```python
from build123d import *

# Parameters (mm, degrees)
BOSS_EXTRUDE1_DEPTH = 3.175
SKETCH2_W           = 156.972
SKETCH2_H           = 22.225
SKETCH2_R           = 4.7625
SKETCH2_R_2         = 0.79375
BOSS_EXTRUDE2_DEPTH = 3.175
FILLET2_R           = 1.27


with BuildPart() as part:
    # Sketch1 → Boss-Extrude1 (new body)
    with BuildSketch(Plane(origin=(0, 0, 0), x_dir=(1, 0, 0), z_dir=(0, 1, 0))):
        Polygon((-78.486, 49.784), (-78.486, 45.72), (-56.261, 45.72), (-56.261, -45.72), (-78.486, -45.72), (-78.486, -49.784), (78.486, -49.784), (78.486, -45.72), (56.261, -45.72), (56.261, 45.72), (78.486, 45.72), (78.486, 49.784), align=None)
    extrude(amount=BOSS_EXTRUDE1_DEPTH)

    # Sketch2 → Boss-Extrude2 (add)
    with BuildSketch(Plane.XY.offset(49.784)):
        with Locations((0, -7.9375)):
            Rectangle(SKETCH2_W, SKETCH2_H)
        with Locations((-67.3735, -7.9375)):
            Circle(SKETCH2_R, mode=Mode.SUBTRACT)
        with Locations(Location((67.3735, -7.9375, 0), (0, 0, 180))):
            Circle(SKETCH2_R, mode=Mode.SUBTRACT)
        with Locations((-47.0535, -12.7)):
            Circle(SKETCH2_R_2, mode=Mode.SUBTRACT)
        with Locations((-37.5285, -12.7)):
            Circle(SKETCH2_R_2, mode=Mode.SUBTRACT)
        with Locations(Location((37.5285, -12.7, 0), (0, 0, 180))):
            Circle(SKETCH2_R_2, mode=Mode.SUBTRACT)
        with Locations(Location((47.0535, -12.7, 0), (0, 0, 180))):
            Circle(SKETCH2_R_2, mode=Mode.SUBTRACT)
    boss_extrude2 = extrude(amount=-BOSS_EXTRUDE2_DEPTH)

    # Mirror2: Boss-Extrude2 across plane
    add(boss_extrude2.mirror(Plane.XY))

    # Fillet2
    # the kernel refuses this fillet: 1.27 mm, written as the material it takes off along each edge
    with BuildSketch(Plane(origin=(-56.261, 0, 45.72), x_dir=(0, 1, 0), z_dir=(-1, 0, 0)), Plane(origin=(56.261, 0, -45.72), x_dir=(0, 1, 0), z_dir=(1, 0, 0)), Plane(origin=(81.514756964, 0, 45.72), x_dir=(0, 1, 0), z_dir=(-1, 0, 0))) as fillet2_piece_1:
        with BuildLine():
            CenterArc((1.211502786, -1.27), FILLET2_R, 90, 72.542396876)
            Line((0, -0.889), (-0.024230056, -0.88138))
            ThreePointArc((-0.024230056, -0.88138), (-0.0254, -0.4445), (-0.0254, 0))
            Line((-0.0254, 0), (0, 0.0254))
            Line((0, 0.0254), (1.211502786, 0.0254))
            Line((1.211502786, 0.0254), (1.211502786, 0))
        make_face()
    extrude(amount=25.253756964, mode=Mode.SUBTRACT)
    with BuildSketch(Plane(origin=(-81.514756964, 0, -45.72), x_dir=(0, 0, -1), z_dir=(1, 0, 0))) as fillet2_piece_2:
        with BuildLine():
            CenterArc((1.27, 1.211502786), FILLET2_R, 180, 72.542396876)
            Line((0, 1.211502786), (-0.0254, 1.211502786))
            Line((-0.0254, 1.211502786), (-0.0254, 0))
            Line((-0.0254, 0), (0, -0.0254))
            ThreePointArc((0, -0.0254), (0.4445, -0.0254), (0.88138, -0.024230056))
            Line((0.88138, -0.024230056), (0.889, 0))
        make_face()
    extrude(amount=25.253756964, mode=Mode.SUBTRACT)
    with BuildSketch(Plane(origin=(81.661, 3.175, 45.72), x_dir=(0, -1, 0), z_dir=(-1, 0, 0)), Plane(origin=(56.261, 3.175, -45.72), x_dir=(0, -1, 0), z_dir=(1, 0, 0)), Plane(origin=(-81.661, 3.175, -45.72), x_dir=(0, -1, 0), z_dir=(1, 0, 0)), Plane(origin=(-56.261, 3.175, 45.72), x_dir=(0, -1, 0), z_dir=(-1, 0, 0))) as fillet2_piece_3:
        with BuildLine():
            CenterArc((FILLET2_R, FILLET2_R), FILLET2_R, 180, 90)
            Line((0, FILLET2_R), (-FILLET2_R * 0.02, FILLET2_R))
            Line((-FILLET2_R * 0.02, FILLET2_R), (-FILLET2_R * 0.02, -FILLET2_R * 0.02))
            Line((-FILLET2_R * 0.02, -FILLET2_R * 0.02), (FILLET2_R, -FILLET2_R * 0.02))
            Line((FILLET2_R, -FILLET2_R * 0.02), (FILLET2_R, 0))
        make_face()
    extrude(amount=25.4, mode=Mode.SUBTRACT)
    with BuildSketch(Plane(origin=(-81.661, -19.05, -46.609), x_dir=(0, 0, -1), z_dir=(1, 0, 0)), Plane(origin=(-81.661, -19.05, -49.784), x_dir=(0, 1, 0), z_dir=(1, 0, 0)), Plane(origin=(-81.661, 3.175, 49.784), x_dir=(0, -1, 0), z_dir=(1, 0, 0)), Plane(origin=(81.661, 3.175, -49.784), x_dir=(0, -1, 0), z_dir=(-1, 0, 0))) as fillet2_piece_4:
        with BuildLine():
            CenterArc((FILLET2_R, FILLET2_R), FILLET2_R, 180, 90)
            Line((0, FILLET2_R), (-FILLET2_R * 0.02, FILLET2_R))
            Line((-FILLET2_R * 0.02, FILLET2_R), (-FILLET2_R * 0.02, -FILLET2_R * 0.02))
            Line((-FILLET2_R * 0.02, -FILLET2_R * 0.02), (FILLET2_R, -FILLET2_R * 0.02))
            Line((FILLET2_R, -FILLET2_R * 0.02), (FILLET2_R, 0))
        make_face()
    extrude(amount=163.322, mode=Mode.SUBTRACT)
    with BuildSketch(Plane(origin=(-81.661, -19.05, 46.609), x_dir=(0, 0, 1), z_dir=(1, 0, 0)), Plane(origin=(-81.661, -19.05, 49.784), x_dir=(0, 1, 0), z_dir=(1, 0, 0))) as fillet2_piece_5:
        with BuildLine():
            CenterArc((FILLET2_R, -FILLET2_R), FILLET2_R, 90, 90)
            Line((0, -FILLET2_R), (-FILLET2_R * 0.02, -FILLET2_R))
            Line((-FILLET2_R * 0.02, -FILLET2_R), (-FILLET2_R * 0.02, FILLET2_R * 0.02))
            Line((-FILLET2_R * 0.02, FILLET2_R * 0.02), (FILLET2_R, FILLET2_R * 0.02))
            Line((FILLET2_R, FILLET2_R * 0.02), (FILLET2_R, 0))
        make_face()
    extrude(amount=163.322, mode=Mode.SUBTRACT)


solid = part.part
```
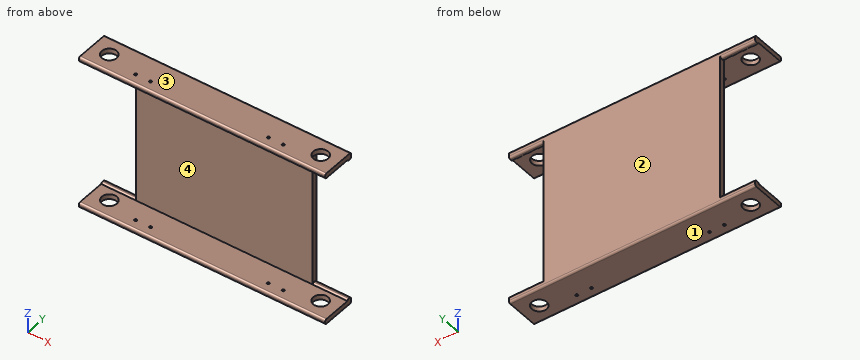
Geometry: final body of the model. Coordinates: model frame, mm. Face numbers are marked on the shaded views. Coordinates: 2 decimals unless noted, no trailing zeros. Order: outer loops, then holes, each group sorted by start corner. A loop starts at its lowest first (then second) coordinate and runs counter-clockwise, first axis right, second up. Notation, with made-up numbers: (22.25, 34.5) -> (51.25, 34.5) arc R13 ccw to (51.25, 46.5) -> close; hole circle Ø6 at (-16, 8.5). An arc over 180 degrees is marked (long way). Write each question's results on one line, items separated by ' | '. Start each with the question number.
1) Cut plane A-A, the plane x = -22.5. Output: boundary loops of the cut face in (y, z) (3 decimals), and give its area (3 significant figures).
2) Mould query, pull axis Z, two halves, no side actions, for the marked faces 1, 2, 3 and 4. Classes: released by +Z, released by -Z, zero draft, split by the parting line, or undercut.
3) Cut plane B-B, the plane z = 7.5. Output: boundary loops of the cut face in (x, y) (3 decimals).
4) Material intervals for line 1 along Z through (x, y) = (28.5, -2); line 2 along Y through (x, z) = (-3.5, -18) (3 decimals); line 3 along Z through (x, y) = (40, 2), sorted ascending.
5) First-contact query: pin 1 (1 mm diameter, centred on x = 37.53, y = -12.7, fed in from +Z); pin 2 (1.6 mm diameter, centred on y = 1.5, z = -4, fed in from +X); pin 3 (10 mm diameter, centred on y = -3.5, z = 38.5, fed in from -X); pin 4 (10 mm diameter, centred on x = -25.5, z = -37, fed in from -Y). Flat tips, straight axial feed; report the tip coordinate or a pass-through.
Checks:
1) outline: (-19.05, -48.514) arc R1.27 ccw to (-17.78, -49.784) -> (1.905, -49.784) arc R1.27 ccw to (3.175, -48.514) -> (3.175, 48.514) arc R1.27 ccw to (1.905, 49.784) -> (-17.78, 49.784) arc R1.27 ccw to (-19.05, 48.514) -> (-19.05, 47.879) arc R1.27 ccw to (-17.78, 46.609) -> (0, 46.609) -> (0, -46.609) -> (-17.78, -46.609) arc R1.27 ccw to (-19.05, -47.879) -> close | area: 435 mm^2
2) face 1: released by -Z | face 2: zero draft | face 3: released by +Z | face 4: undercut
3) outline: (-56.261, 0) -> (56.261, 0) -> (56.261, 3.175) -> (-56.261, 3.175) -> close
4) line 1: -49.78 to -46.61, 46.61 to 49.78 | line 2: 0 to 3.175 | line 3: -49.78 to 49.78
5) pin 1: through | pin 2: x = 56.26 | pin 3: x = -56.26 | pin 4: y = 0
